```python
from build123d import *

# Parameters (mm, degrees)
BOSS_EXTRU_1_DEPTH         = 3
BOSS_EXTRU_2_DEPTH         = 100
R_P_TITION_LIN_AIRE1_COUNT = 2
R_P_TITION_LIN_AIRE1_PITCH = 103
ESQUISSE5_W                = 2.97567345
ESQUISSE5_H                = 100
BOSS_EXTRU_3_DEPTH         = 137
ESQUISSE6_W                = 2.705773981
ESQUISSE6_H                = 100
ESQUISSE9_R                = 1.462141601
ENL_V_MAT_EXTRU_8_DEPTH    = 10
ENL_V_MAT_EXTRU_10_DEPTH   = 10


with BuildPart() as part:
    # Esquisse2 → Boss.-Extru.1 (new body)
    with BuildSketch(Plane.XY):
        Polygon((0, 0), (0, 140), (3.942801894, 140), (47.364817767, 98.480775301), (30, 0), align=None)
    boss_extru_1 = extrude(amount=BOSS_EXTRU_1_DEPTH)

    # Esquisse4 → Boss.-Extru.2 (add)
    with BuildSketch(Plane.XY.offset(3)):
        Polygon((0, 0), (0, 3.006117571), (30.530059635, 3.006117571), (30, 0), align=None)
    extrude(amount=BOSS_EXTRU_2_DEPTH)

    # Répétition linéaire1: Boss.-Extru.1 ×2
    with Locations(*[(0, 0, i * R_P_TITION_LIN_AIRE1_PITCH) for i in range(1, R_P_TITION_LIN_AIRE1_COUNT)]):
        add(boss_extru_1)

    # Esquisse5 → Boss.-Extru.3 (add)
    with BuildSketch(Plane(origin=(0, 3.006117571, 0), x_dir=(1, 0, 0), z_dir=(0, 1, 0))):
        with Locations((1.487836725, -53)):
            Rectangle(ESQUISSE5_W, ESQUISSE5_H)
    extrude(amount=BOSS_EXTRU_3_DEPTH)

    # Balayage1: sweep along a curve in space
    with BuildLine() as balayage1_path:
        Line((30.530059635, 3.006117571, 103), (47.364817767, 98.480775301, 103))
    # Esquisse6 → Balayage1 (sweep)
    with BuildSketch(Plane(origin=(0, 3.006117571, 0), x_dir=(1, 0, 0), z_dir=(0, 1, 0))):
        with Locations((29.177172645, -53)):
            Rectangle(ESQUISSE6_W, ESQUISSE6_H)
    sweep(path=balayage1_path.line)

    # Esquisse9 → Enlèv. mat.-Extru.8 (cut)
    with BuildSketch(Plane(origin=(2.97567345, 0, 0), x_dir=(0, 0, -1), z_dir=(1, 0, 0))):
        with Locations((-80, 110)):
            Circle(ESQUISSE9_R)
    enl_v_mat_extru_8 = extrude(amount=-ENL_V_MAT_EXTRU_8_DEPTH, mode=Mode.SUBTRACT)

    # Symétrie3: Enlèv. mat.-Extru.8 across plane
    add(enl_v_mat_extru_8.mirror(Plane.XY.offset(53)), mode=Mode.SUBTRACT)

    # Esquisse11 → Enlèv. mat.-Extru.10 (cut)
    with BuildSketch(Plane(origin=(29.095389312, -5.13030215, 0), x_dir=(0, 0, -1), z_dir=(0.9848077530122089, -0.17364817766692642, 0))):
        Polygon((-6.160430803, 48.968309083), (-6.160430803, 95.489627834), (-34.939480046, 62.478304571), (-34.939480046, 15.95698582), align=None)
    enl_v_mat_extru_10 = extrude(amount=-ENL_V_MAT_EXTRU_10_DEPTH, mode=Mode.SUBTRACT)

    # Symétrie4: Enlèv. mat.-Extru.10 across plane
    add(enl_v_mat_extru_10.mirror(Plane.XY.offset(53)), mode=Mode.SUBTRACT)


solid = part.part
```
Geometry: final body of the model. Coordinates: model frame, mm. A direction names the side the tool comes from. Coordinates: 2 decimals unless noted, no trailing zeros. Order: outer loops, then holes, each group sorted by start corner. A loop starts at its lowest first (then second) coordinate and runs counter-clockwise, first axis right, second up. Notation, with made-up numbers: (-33.75, 32.25) -> (19.25, 32.25) arc R23 ccw to (19.25, 45.25) -> close; hole circle Ø1 at (-38.75, 3.25). An arc over 180 degrees is marked (long way). Write item = value, one per line.
(1) Cut plane A-A on z = 45.5. Return loops of the section in (x, y), plus the area to 3 significant figures.
Solved:
outline = (0, 0) -> (30, 0) -> (47.36, 98.48) -> (44.66, 98.48) -> (27.82, 3.01) -> (2.98, 3.01) -> (2.98, 140.01) -> (0, 140.01) -> close
area = 757 mm²
(2) Cut plane B-B on y = 22.5. Return loops of the section in (x, z), plus the area to 3 significant figures.
Solved:
outline = (0, 0) -> (33.97, 0) -> (33.97, 24.39) -> (31.26, 24.8) -> (31.26, 3) -> (2.98, 3) -> (2.98, 103) -> (31.26, 103) -> (31.26, 81.2) -> (33.97, 81.61) -> (33.97, 106) -> (0, 106) -> close; (31.26, 34.94) -> (33.97, 34.94) -> (33.97, 71.06) -> (31.26, 71.06) -> close
area = 716 mm²
(3) Cut plane C-C on z = 83. Return loops of the section in (x, y), plus the area to 3 significant figures.
Solved:
outline = (0, 0) -> (30, 0) -> (34.24, 24.07) -> (31.62, 24.53) -> (27.82, 3.01) -> (2.98, 3.01) -> (2.98, 140.01) -> (0, 140.01) -> close; (39.7, 70.35) -> (42.32, 69.89) -> (47.36, 98.48) -> (44.66, 98.48) -> close
area = 633 mm²
(4) Line query: line 1 (Z direction, x = 2.1, y = 110); line 2 (Z direction, x = 19, y = 29.5); line 3 (Y direction, x = 1.75, z = 80). Output: solid intervals per line, ascending.
Solved:
line_1 = 0 to 24.54, 27.46 to 78.54, 81.46 to 106
line_2 = 0 to 3, 103 to 106
line_3 = 0 to 108.54, 111.46 to 140.01
(5) Pin query (flat end, axial travel): pin 1 Ø1.5 at (x, y) = (28.5, 36.5) entering from -Z; pin 2 Ø4 at (y, z) = (50, 90) entering from +X; pin 3 Ø2 at (x, z) = (45.5, 35) entering from +Y; pin 4 Ø1 at (x, z) = (8.5, 47) entering from +Y. Return the tip coordinate at first contact, or that it passes through.
Solved:
pin_1 = 0
pin_2 = 2.98
pin_3 = 98.48
pin_4 = 3.01
(6) Cut plane D-D on y = 110. Return loops of the section in (x, z), plus the area to 3 significant figures.
Solved:
outline = (0, 0) -> (35.32, 0) -> (35.32, 3) -> (2.98, 3) -> (2.98, 24.54) -> (0, 24.54) -> close; (0, 27.46) -> (2.98, 27.46) -> (2.98, 78.54) -> (0, 78.54) -> close; (0, 81.46) -> (2.98, 81.46) -> (2.98, 103) -> (35.32, 103) -> (35.32, 106) -> (0, 106) -> close
area = 492 mm²
(7) Pull-direction query (X, two-part tool) for faces 4 (the flat face through (33.4, 26.84, 85.25)), 5 (the flat face through (21, 72, 103)), 6 (the cylindrical face through (1.51, 108.7, 79.33)); classes: pulls with the +X half, pulls with the -X half, needs draft (parallel to the pull), parting line crosses it, or undercut.
Solved:
face_4 = pulls with the +X half
face_5 = undercut
face_6 = needs draft
(8) Access query for faces 1 (the flat face through (21, 72, 3)), 2 (the flat face through (41.56, 73.11, 85.65)), 3 (the flat face through (33.4, 26.84, 20.75)). Directions: +Z, -Z, +X, -X, +Y, -Y. A direction counts if a zero-diameter tool reaches every point of the face in a straight line with its end or side. Return the directions, or none.
Solved:
face_1 = +Y
face_2 = -Y
face_3 = +X, +Y
